from build123d import *

# Parameters (mm, degrees)
SKETCH1_W            = 60
SKETCH1_H            = 30
BOSS_EXTRUDE1_DEPTH  = 5
SKETCH2_W            = 35
SKETCH2_H            = 30
BOSS_EXTRUDE2_DEPTH  = 15
SKETCH4_R            = 11
CUT_EXTRUDE1_DEPTH   = 48.5
M3_CLEARANCE_HOLE1_D = 3.4
FILLET1_R            = 1
FILLET2_R            = 1
FILLET3_R            = 1
FILLET4_R            = 1


with BuildPart() as part:
    # Sketch1 → Boss-Extrude1 (new body)
    with BuildSketch(Plane(origin=(0, 0, 0), x_dir=(1, 0, 0), z_dir=(0, 1, 0))):
        with Locations((12.386363636, 4.042207792)):
            Rectangle(SKETCH1_W, SKETCH1_H)
    extrude(amount=BOSS_EXTRUDE1_DEPTH)

    # Sketch2 → Boss-Extrude2 (add)
    with BuildSketch(Plane(origin=(0, 5, 0), x_dir=(1, 0, 0), z_dir=(0, 1, 0))):
        with Locations((12.386363636, 4.042207792)):
            Rectangle(SKETCH2_W, SKETCH2_H)
    extrude(amount=BOSS_EXTRUDE2_DEPTH)

    # Sketch4 → Cut-Extrude1 (cut, through all)
    with BuildSketch(Plane(origin=(29.886363636, 0, 0), x_dir=(0, 0, -1), z_dir=(1, 0, 0))):
        with Locations((4.042207792, 20)):
            Circle(SKETCH4_R)
    extrude(amount=-CUT_EXTRUDE1_DEPTH, mode=Mode.SUBTRACT)

    # M3 Clearance Hole1 (through all)
    with Locations(Plane(origin=(0, 5, 0), x_dir=(1, 0, 0), z_dir=(0, 1, 0))):
        with Locations((36.136363636, 4.042207792), (-11.363636364, 4.042207792)):
            Hole(M3_CLEARANCE_HOLE1_D / 2)

    # Fillet1
    fillet1_edges = [part.edges().sort_by_distance(p)[0] for p in [
        (12.386363636, 20, 10.957792208),
    ]]
    fillet(fillet1_edges, radius=FILLET1_R)

    # Fillet2
    fillet2_edges = [part.edges().sort_by_distance(p)[0] for p in [
        (12.386363636, 20, -19.042207792),
    ]]
    fillet(fillet2_edges, radius=FILLET2_R)

    # Fillet3
    fillet3_edges = [part.edges().sort_by_distance(p)[0] for p in [
        (42.386363636, 5, -4.042207792),
    ]]
    fillet(fillet3_edges, radius=FILLET3_R)

    # Fillet4
    fillet4_edges = [part.edges().sort_by_distance(p)[0] for p in [
        (-17.613636364, 5, -4.042207792),
    ]]
    fillet(fillet4_edges, radius=FILLET4_R)


solid = part.part
Verification items for the finished model (mm, model axes). A direction names the side the tool comes from. Give positions to 0.01 mm unless a question says otherwise; leave off trailing zeros. Loops run counter-clockwise (first coordinate to the right, second up) from the corner with the lowest first, then second, coordinate; pieces in that order, holes last. Notation, with made-up numbers: (87.25, 71) - (126.25, 71) arc R6 cw to (126.25, 80) - close; hole circle Ø11 at (25, 0). An arc over 180 degrees is marked (long way). Write item = value, one per line. Start each with the question number.
Q1. Thickness scan on line 1 (Y direction, x = 36, z = 4.25); line 2 (X direction, y = 7.25, z = -5.5); line 3 (Z direction, x = -3.5, y = 11.25). Record the ranges inside material, lowest first.
Q2. Cross-section at A-A, the plane y = 17.25. Enter the section's corners in (x, z), and give its area (3 significant figures).
Q3. Depth check by flat-ended pin: P1, Ø2, axis at x = -11.36, z = -4.04, coming from the -Y side; P2, Ø6, axis at x = 38, z = -11, coming from the +Y side; P3, Ø4.5, axis at y = 11.5, z = -0.5, coming from the -X side. Enter the tip coordinate at first touch or a pass-through.
Q4. Tool access check on faces 5 (the face through (12, 20, -17)), 6 (the face through (-5.114, 7, -4)), 7 (the face through (34, 5, -4)). Record the directions out of +Z, -Z, +X, -X, +Y, -Y that give a thin tool (end or side, any length) a straight path to the whole face; none if there is none.
Q5. Cross-section at B-B, the plane x = 4. Enter the section's corners in (y, z).
Q6. Cross-section at D-D, the plane y = 14.5. Enter the section's corners in (x, z), and give its area (3 significant figures).
Q7. Mould release check, pull along Z, two halves, no side actions. Record for faces 1 (the face through (-10.015, 2.465, -3.008)), 2 (the face through (37.835, 2.465, -4.117)), 3 (the face through (-8, 5, -4)), 4 (the face through (12, 7, -19.042)): released by +Z, released by -Z, zero draft, split by the parting line, or undercut.
Q8. Cross-section at C-C, the plane z = -12.5. Enter the section's corners in (x, y).
Answer key:
q1.line_1 = 0 to 5
q1.line_2 = -5.11 to 29.89
q1.line_3 = -19.04 to -10.71, 2.62 to 10.96
q2.outline = (-5.11, -19.04) - (29.89, -19.04) - (29.89, -14.69) - (-5.11, -14.69) - close; (-5.11, 6.61) - (29.89, 6.61) - (29.89, 10.96) - (-5.11, 10.96) - close
q2.area = 304 mm^2
q3.P1 = through
q3.P2 = 5
q3.P3 = -5.11
q4.face_5 = +Z, -Z, +X, -X, +Y
q4.face_6 = +Z, -Z, -X, +Y
q4.face_7 = +Z, -Z, +X, +Y
q5.outline = (0, -19.04) - (19, -19.04) arc R1 ccw to (20, -18.04) - (20, -15.04) arc R11 cw to (20, 6.96) - (20, 9.96) arc R1 ccw to (19, 10.96) - (0, 10.96) - close
q6.outline = (-5.11, -19.04) - (29.89, -19.04) - (29.89, -13.57) - (-5.11, -13.57) - close; (-5.11, 5.48) - (29.89, 5.48) - (29.89, 10.96) - (-5.11, 10.96) - close
q6.area = 383 mm^2
q7.face_1 = undercut
q7.face_2 = undercut
q7.face_3 = zero draft
q7.face_4 = released by -Z
q8.outline = (-17.61, 0) - (42.39, 0) - (42.39, 4) arc R1 ccw to (41.39, 5) - (29.89, 5) - (29.89, 12.97) - (-5.11, 12.97) - (-5.11, 5) - (-16.61, 5) arc R1 ccw to (-17.61, 4) - close
